For this review, take the finished solid that the model builds, in its own axes (mm). Give positions to 0.01 mm unless a question says otherwise; leave off trailing zeros. Order: outer loops, then holes, each group sorted by start corner. A loop starts at its lowest first (then second) coordinate and runs counter-clockwise, first axis right, second up.
Item 1: Consider section B-B (z = -0.55). Give the number of separate pieces and of enclosed holes in the cut face, plus the area to 3 significant figures.
Item 2: Consider section A-A (y = 13.63). Give the boundary of the cut face in (x, z).
Item 3: For probe 1 along Y at (x, z) = (-9.8, -0.5); probe 2 along Y at (x, z) = (9.5, -0.1), list the stretches that pass through material, from the lowest coordinate up.
Item 4: Consider section C-C (x = -10.5). Give the boundary of the cut face in (y, z).
```python
from build123d import *

# Parameters (mm, degrees)
SKETCH012_R                             = 1.6
PAD006_DEPTH                            = 1
SKETCH019_R                             = 0.5
POCKET003_DEPTH                         = 86.464442
POCKET003_DEPTH_BACK                    = 85.464442
SKETCH019_LINEARPATTERN001_2_R          = 0.5
POCKET003_LINEARPATTERN001_2_DEPTH      = 86.464442
POCKET003_LINEARPATTERN001_2_DEPTH_BACK = 85.464442
SKETCH019_LINEARPATTERN001_3_R          = 0.5
POCKET003_LINEARPATTERN001_3_DEPTH      = 86.464442
POCKET003_LINEARPATTERN001_3_DEPTH_BACK = 85.464442
SKETCH019_LINEARPATTERN001_4_R          = 0.5
POCKET003_LINEARPATTERN001_4_DEPTH      = 86.464442
POCKET003_LINEARPATTERN001_4_DEPTH_BACK = 85.464442
SKETCH019_LINEARPATTERN001_5_R          = 0.5
POCKET003_LINEARPATTERN001_5_DEPTH      = 86.464442
POCKET003_LINEARPATTERN001_5_DEPTH_BACK = 85.464442
SKETCH019_LINEARPATTERN001_6_R          = 0.5
POCKET003_LINEARPATTERN001_6_DEPTH      = 86.464442
POCKET003_LINEARPATTERN001_6_DEPTH_BACK = 85.464442
SKETCH019_LINEARPATTERN001_7_R          = 0.5
POCKET003_LINEARPATTERN001_7_DEPTH      = 86.464442
POCKET003_LINEARPATTERN001_7_DEPTH_BACK = 85.464442
SKETCH019_LINEARPATTERN001_8_R          = 0.5
POCKET003_LINEARPATTERN001_8_DEPTH      = 86.464442
POCKET003_LINEARPATTERN001_8_DEPTH_BACK = 85.464442
SKETCH019_LINEARPATTERN001_9_R          = 0.5
POCKET003_LINEARPATTERN001_9_DEPTH      = 86.464442
POCKET003_LINEARPATTERN001_9_DEPTH_BACK = 85.464442


with BuildPart() as part:
    # Sketch012 → Pad006 (new body)
    with BuildSketch(Plane.XY):
        with BuildLine():
            Line((9.8, 17.1), (-9.8, 17.1))
            ThreePointArc((-9.8, 17.1), (-11.92132, 16.22132), (-12.8, 14.1))
            Line((-12.8, 14.1), (-12.8, -17.1))
            Line((-12.8, -17.1), (12.8, -17.1))
            Line((12.8, -17.1), (12.8, 14.1))
            ThreePointArc((12.8, 14.1), (11.92132, 16.22132), (9.8, 17.1))
        make_face()
        with Locations((-9.8, 14.1)):
            Circle(SKETCH012_R, mode=Mode.SUBTRACT)
        with Locations((9.8, -14.1)):
            Circle(SKETCH012_R, mode=Mode.SUBTRACT)
    extrude(amount=-PAD006_DEPTH)

    # Sketch019 → Pocket003 (cut, two sides)
    with BuildSketch(Plane.XY) as pocket003_sk:
        with Locations((11.45, -11.09)):
            Circle(SKETCH019_R)
    pocket003 = extrude(amount=-POCKET003_DEPTH, mode=Mode.SUBTRACT) + extrude(pocket003_sk.sketch, amount=POCKET003_DEPTH_BACK, mode=Mode.SUBTRACT)

    # Sketch019 LinearPattern001 2 → Pocket003 LinearPattern001 2 (cut, two sides)
    with BuildSketch(Plane(origin=(0, 2.54, 0), x_dir=(1, 0, 0), z_dir=(0, 0, 1))) as pocket003_linearpattern001_2_sk:
        with Locations((11.45, -11.09)):
            Circle(SKETCH019_LINEARPATTERN001_2_R)
    pocket003_linearpattern001_2 = extrude(amount=-POCKET003_LINEARPATTERN001_2_DEPTH, mode=Mode.SUBTRACT) + extrude(pocket003_linearpattern001_2_sk.sketch, amount=POCKET003_LINEARPATTERN001_2_DEPTH_BACK, mode=Mode.SUBTRACT)

    # Sketch019 LinearPattern001 3 → Pocket003 LinearPattern001 3 (cut, two sides)
    with BuildSketch(Plane(origin=(0, 5.08, 0), x_dir=(1, 0, 0), z_dir=(0, 0, 1))) as pocket003_linearpattern001_3_sk:
        with Locations((11.45, -11.09)):
            Circle(SKETCH019_LINEARPATTERN001_3_R)
    pocket003_linearpattern001_3 = extrude(amount=-POCKET003_LINEARPATTERN001_3_DEPTH, mode=Mode.SUBTRACT) + extrude(pocket003_linearpattern001_3_sk.sketch, amount=POCKET003_LINEARPATTERN001_3_DEPTH_BACK, mode=Mode.SUBTRACT)

    # Sketch019 LinearPattern001 4 → Pocket003 LinearPattern001 4 (cut, two sides)
    with BuildSketch(Plane(origin=(0, 7.62, 0), x_dir=(1, 0, 0), z_dir=(0, 0, 1))) as pocket003_linearpattern001_4_sk:
        with Locations((11.45, -11.09)):
            Circle(SKETCH019_LINEARPATTERN001_4_R)
    pocket003_linearpattern001_4 = extrude(amount=-POCKET003_LINEARPATTERN001_4_DEPTH, mode=Mode.SUBTRACT) + extrude(pocket003_linearpattern001_4_sk.sketch, amount=POCKET003_LINEARPATTERN001_4_DEPTH_BACK, mode=Mode.SUBTRACT)

    # Sketch019 LinearPattern001 5 → Pocket003 LinearPattern001 5 (cut, two sides)
    with BuildSketch(Plane(origin=(0, 10.16, 0), x_dir=(1, 0, 0), z_dir=(0, 0, 1))) as pocket003_linearpattern001_5_sk:
        with Locations((11.45, -11.09)):
            Circle(SKETCH019_LINEARPATTERN001_5_R)
    pocket003_linearpattern001_5 = extrude(amount=-POCKET003_LINEARPATTERN001_5_DEPTH, mode=Mode.SUBTRACT) + extrude(pocket003_linearpattern001_5_sk.sketch, amount=POCKET003_LINEARPATTERN001_5_DEPTH_BACK, mode=Mode.SUBTRACT)

    # Sketch019 LinearPattern001 6 → Pocket003 LinearPattern001 6 (cut, two sides)
    with BuildSketch(Plane(origin=(0, 12.7, 0), x_dir=(1, 0, 0), z_dir=(0, 0, 1))) as pocket003_linearpattern001_6_sk:
        with Locations((11.45, -11.09)):
            Circle(SKETCH019_LINEARPATTERN001_6_R)
    pocket003_linearpattern001_6 = extrude(amount=-POCKET003_LINEARPATTERN001_6_DEPTH, mode=Mode.SUBTRACT) + extrude(pocket003_linearpattern001_6_sk.sketch, amount=POCKET003_LINEARPATTERN001_6_DEPTH_BACK, mode=Mode.SUBTRACT)

    # Sketch019 LinearPattern001 7 → Pocket003 LinearPattern001 7 (cut, two sides)
    with BuildSketch(Plane(origin=(0, 15.24, 0), x_dir=(1, 0, 0), z_dir=(0, 0, 1))) as pocket003_linearpattern001_7_sk:
        with Locations((11.45, -11.09)):
            Circle(SKETCH019_LINEARPATTERN001_7_R)
    pocket003_linearpattern001_7 = extrude(amount=-POCKET003_LINEARPATTERN001_7_DEPTH, mode=Mode.SUBTRACT) + extrude(pocket003_linearpattern001_7_sk.sketch, amount=POCKET003_LINEARPATTERN001_7_DEPTH_BACK, mode=Mode.SUBTRACT)

    # Sketch019 LinearPattern001 8 → Pocket003 LinearPattern001 8 (cut, two sides)
    with BuildSketch(Plane(origin=(0, 17.78, 0), x_dir=(1, 0, 0), z_dir=(0, 0, 1))) as pocket003_linearpattern001_8_sk:
        with Locations((11.45, -11.09)):
            Circle(SKETCH019_LINEARPATTERN001_8_R)
    pocket003_linearpattern001_8 = extrude(amount=-POCKET003_LINEARPATTERN001_8_DEPTH, mode=Mode.SUBTRACT) + extrude(pocket003_linearpattern001_8_sk.sketch, amount=POCKET003_LINEARPATTERN001_8_DEPTH_BACK, mode=Mode.SUBTRACT)

    # Sketch019 LinearPattern001 9 → Pocket003 LinearPattern001 9 (cut, two sides)
    with BuildSketch(Plane(origin=(0, 20.32, 0), x_dir=(1, 0, 0), z_dir=(0, 0, 1))) as pocket003_linearpattern001_9_sk:
        with Locations((11.45, -11.09)):
            Circle(SKETCH019_LINEARPATTERN001_9_R)
    pocket003_linearpattern001_9 = extrude(amount=-POCKET003_LINEARPATTERN001_9_DEPTH, mode=Mode.SUBTRACT) + extrude(pocket003_linearpattern001_9_sk.sketch, amount=POCKET003_LINEARPATTERN001_9_DEPTH_BACK, mode=Mode.SUBTRACT)

    # Mirrored004: Pocket003, Pocket003 LinearPattern001 2, Pocket003 LinearPattern001 3, Pocket003 LinearPattern001 4, Pocket003 LinearPattern001 5, Pocket003 LinearPattern001 6, Pocket003 LinearPattern001 7, Pocket003 LinearPattern001 8, Pocket003 LinearPattern001 9 across YZ
    add(pocket003.mirror(Plane.YZ), mode=Mode.SUBTRACT)
    add(pocket003_linearpattern001_2.mirror(Plane.YZ), mode=Mode.SUBTRACT)
    add(pocket003_linearpattern001_3.mirror(Plane.YZ), mode=Mode.SUBTRACT)
    add(pocket003_linearpattern001_4.mirror(Plane.YZ), mode=Mode.SUBTRACT)
    add(pocket003_linearpattern001_5.mirror(Plane.YZ), mode=Mode.SUBTRACT)
    add(pocket003_linearpattern001_6.mirror(Plane.YZ), mode=Mode.SUBTRACT)
    add(pocket003_linearpattern001_7.mirror(Plane.YZ), mode=Mode.SUBTRACT)
    add(pocket003_linearpattern001_8.mirror(Plane.YZ), mode=Mode.SUBTRACT)
    add(pocket003_linearpattern001_9.mirror(Plane.YZ), mode=Mode.SUBTRACT)


with BuildPart() as part_1:
    # Body005 placement: moved
    add(part.part.moved(Location((0, 17.1, 0))))


solid = part_1.part
```
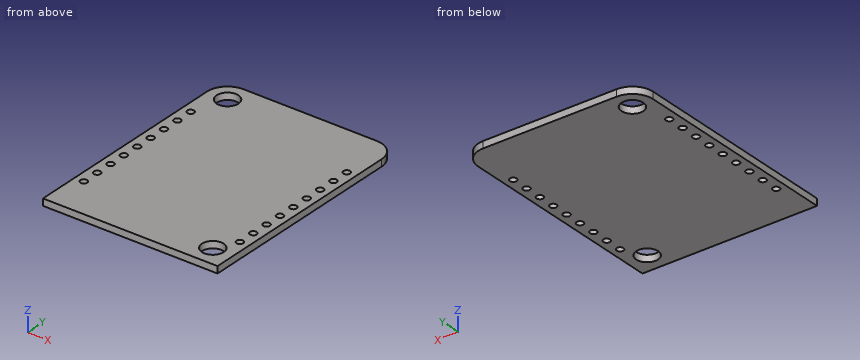
Resolved:
1. separate pieces: 1
1. enclosed holes: 20
1. area: 841 mm2
2. outline: (-12.8, -1) - (-11.95, -1) - (-11.95, 0) - (-12.8, 0) - close; (-10.95, -1) - (10.95, -1) - (10.95, 0) - (-10.95, 0) - close; (11.95, -1) - (12.8, -1) - (12.8, 0) - (11.95, 0) - close
3. probe 1: y = 0 to 29.6, 32.8 to 34.2
3. probe 2: y = 0 to 1.43, 4.57 to 34.2
4. outline: (0, -1) - (29.76, -1) - (29.76, 0) - (0, 0) - close; (32.64, -1) - (34.12, -1) - (34.12, 0) - (32.64, 0) - close
